Work out the finished part from the listing and answer in its coordinate system (mm). Round coordinates to 2 decimals unless told otherwise and drop trailing zeros. Order: outer loops, then holes, each group sorted by start corner. A loop starts at its lowest first (then second) coordinate and runs counter-clockwise, first axis right, second up. Notation, with made-up numbers: (-16.75, 64) - (16.25, 64) arc R21 ccw to (16.25, 101) - close; hole circle Ø6 at (60.25, -21). An arc over 180 degrees is marked (long way). One line per question, with ' | ' between items. Start each with the question number.
from build123d import *

# Parameters (mm, degrees)
BOSS_EXTRU_1_DEPTH = 4.5
CONG_8_R           = 3
CONG_9_R           = 3


with BuildPart() as part:
    # Esquisse1 → Boss.-Extru.1 (new body)
    with BuildSketch(Plane.XY):
        with BuildLine():
            Line((0, 0), (0, 33))
            Line((0, 33), (-17, 33))
            Line((-17, 33), (-7.745966692, -2))
            ThreePointArc((-7.745966692, -2), (-4.186842685, 0.215571991), (0, 0))
        make_face()
    extrude(amount=BOSS_EXTRU_1_DEPTH)

    # Congé8
    cong_8_edges = [part.edges().sort_by_distance(p)[0] for p in [
        (-17, 33, 2.25),
    ]]
    fillet(cong_8_edges, radius=CONG_8_R)

    # Congé9
    cong_9_edges = [part.edges().sort_by_distance(p)[0] for p in [
        (0, 33, 2.25),
    ]]
    fillet(cong_9_edges, radius=CONG_9_R)


solid = part.part
1) Flat-ended cylindrical pins translate along their axes: pin 1 (2 mm diameter, centred on y = 21, z = 4, fed in from -X); pin 2 (6 mm diameter, centred on x = -12.5, y = 9.5, fed in from +Z). Find the tip coordinate at first contact, or state that the pin passes through.
2) Section B-B on y = 7.5 is taken. Give the vertices of the cut face in (x, z).
3) Section C-C on x = -9.25 is taken. Give the vertices of the cut face in (y, z), and give its area (3 significant figures).
4) Section A-A on z = 1.45 is taken. Give the vertices of the cut face in (x, y).
5) Straight lines are drawn through the part: line 1 (Y direction, x = -6.5, z = 3.5); line 2 (X direction, y = 2.5, z = 3.75); line 3 (Y direction, x = -4.75, z = 3.5). For each, find the intervals that lie inside material, in ascending order.
6) Determine the mould class of faces 1 (the flat face through (0, 15, 2)), 2 (the cylindrical face through (-15.46, 31.86, 2.28)), 3 (the flat face through (-8, 33, 2)), 4 (the cylindrical face through (-4.24, 0.2, 2.22)) for opening direction X: released by +X, released by -X, zero draft, split by the parting line, or undercut.
Recorded:
1) pin 1: stops at x = -14.09 | pin 2: stops at z = 4.5
2) outline: (-10.26, 0) - (0, 0) - (0, 4.5) - (-10.26, 4.5) - close
3) outline: (3.69, 0) - (33, 0) - (33, 4.5) - (3.69, 4.5) - close | area: 132 mm²
4) outline: (-16, 29.23) - (-7.75, -2) arc R7 cw to (0, 0) - (0, 30) arc R3 ccw to (-3, 33) - (-13.1, 33) arc R3 ccw to start
5) line 1: y = -0.86 to 33 | line 2: x = -8.94 to 0 | line 3: y = 0.04 to 33
6) face 1: released by +X | face 2: released by -X | face 3: zero draft | face 4: undercut
